Could you check a few things on this model? Use its own coordinates, in mm. Coordinates: 2 decimals unless noted, no trailing zeros. Write each loop counter-clockwise with the first axis right and the second up, starting at its lowest first coordinate (ties: lowest second). Pieces come first, ordered by that corner, then holes. Notation, with made-up numbers: (-12.75, -38) - (35.25, -38) arc R11 cw to (35.25, -22) - close; hole circle Ø7 at (16, 33.25). An arc over 180 degrees is marked (long way). Answer as a JSON object with one key per item and string values. Group by question number.
1) We'd pull the mould along Z, two halves only. Please class faces 1 (the flat face through (79, 3, -71)), 2 (the flat face through (117, 2, -115)), 3 (the flat face through (33, 2, -35)): released by +Z, released by -Z, zero draft, split by the parting line, or undercut.
2) If we section it at B-B (z = -51.5): Write out the boundary of the cut face in (x, y), plus the area to 3 significant figures.
3) Will these pins go through, and if not, where does the flat tip stop? pin 1 Ø1.5 at (y, z) = (1.5, -126) entering from +X; pin 2 Ø1 at (x, y) = (21.5, 1) entering from -Z; pin 3 Ø1.5 at (y, z) = (2, -5.5) entering from -X; pin 4 Ø1.9 at (x, z) = (100, -130) entering from +Y.
4) If we section it at A-A (x = 17): Write out the boundary of the cut face in (y, z), plus the area to 3 significant figures.
5) Please list where these lines run through material, in increasing order: line 1 along X through (y, z) = (2.7, -71.5); line 2 along X through (y, z) = (0.75, -45.5); line 3 along Z through (x, y) = (73, 2.8).
6) If we section it at C-C (y = 2.25): State how many separate pieces and enclosed holes the cut face has, plus the area to 3 significant figures.
```python
from build123d import *

# Parameters (mm, degrees)
SKETCH_1_W          = 130
SKETCH_1_H          = 140
SKETCH_1_R          = 1.6
SKETCH_1_W_2        = 24
SKETCH_1_H_2        = 112
EXTRUDE_1_DEPTH     = 3
SKETCH_2_W          = 25
SKETCH_2_H          = 25
CUT_EXTRUDE_1_DEPTH = 3
SKETCH_3_W          = 40
SKETCH_3_H          = 10
SKETCH_3_W_2        = 15.4
SKETCH_3_H_2        = 20
SKETCH_3_W_3        = 16
SKETCH_3_W_4        = 43.4
SKETCH_3_H_3        = 12
SKETCH_3_W_5        = 10
SKETCH_3_H_4        = 16
CUT_EXTRUDE_2_DEPTH = 192.07328437
FILLET_1_R          = 2


with BuildPart() as part:
    # 草图1 → 凸台-拉伸1 (new body)
    with BuildSketch(Plane(origin=(0, 0, 0), x_dir=(1, 0, 0), z_dir=(0, 1, 0))):
        with Locations((65, 70)):
            Rectangle(SKETCH_1_W, SKETCH_1_H)
        with Locations(Location((98.6, 78.5, 0), (0, 0, 270))):
            Circle(SKETCH_1_R, mode=Mode.SUBTRACT)
        with Locations(Location((80.6, 78.5, 0), (0, 0, 90))):
            Circle(SKETCH_1_R, mode=Mode.SUBTRACT)
        with Locations(Location((98.6, 51.5, 0), (0, 0, 90))):
            Circle(SKETCH_1_R, mode=Mode.SUBTRACT)
        with Locations(Location((80.6, 51.5, 0), (0, 0, 270))):
            Circle(SKETCH_1_R, mode=Mode.SUBTRACT)
        with Locations(Location((127, 85, 0), (0, 0, 270))):
            Circle(SKETCH_1_R, mode=Mode.SUBTRACT)
        with Locations(Location((113, 85, 0), (0, 0, 90))):
            Circle(SKETCH_1_R, mode=Mode.SUBTRACT)
        with Locations(Location((120, 66.4, 0), (0, 0, 270))):
            Circle(SKETCH_1_R, mode=Mode.SUBTRACT)
        with Locations(Location((120, 34.4, 0), (0, 0, 270))):
            Circle(SKETCH_1_R, mode=Mode.SUBTRACT)
        with Locations(Location((10, 34.4, 0), (0, 0, 90))):
            Circle(SKETCH_1_R, mode=Mode.SUBTRACT)
        with Locations(Location((10, 66.4, 0), (0, 0, 90))):
            Circle(SKETCH_1_R, mode=Mode.SUBTRACT)
        with Locations(Location((3, 85, 0), (0, 0, 90))):
            Circle(SKETCH_1_R, mode=Mode.SUBTRACT)
        with Locations(Location((17, 85, 0), (0, 0, 270))):
            Circle(SKETCH_1_R, mode=Mode.SUBTRACT)
        with Locations(Location((30, 130, 0), (0, 0, 270))):
            Circle(SKETCH_1_R, mode=Mode.SUBTRACT)
        with Locations(Location((100, 130, 0), (0, 0, 90))):
            Circle(SKETCH_1_R, mode=Mode.SUBTRACT)
        with Locations(Location((80.4, 82.5, 0), (0, 0, 270))):
            Circle(SKETCH_1_R, mode=Mode.SUBTRACT)
        with Locations(Location((80.4, 47.5, 0), (0, 0, 90))):
            Circle(SKETCH_1_R, mode=Mode.SUBTRACT)
        with Locations(Location((102.4, 82.5, 0), (0, 0, 270))):
            Circle(SKETCH_1_R, mode=Mode.SUBTRACT)
        with Locations(Location((102.4, 47.5, 0), (0, 0, 90))):
            Circle(SKETCH_1_R, mode=Mode.SUBTRACT)
        with Locations((65, 65)):
            Rectangle(SKETCH_1_W_2, SKETCH_1_H_2, mode=Mode.SUBTRACT)
    extrude(amount=EXTRUDE_1_DEPTH)

    # 草图2 → 切除-拉伸1 (cut)
    with BuildSketch(Plane(origin=(0, 3, 0), x_dir=(1, 0, 0), z_dir=(0, 1, 0))):
        with Locations((12.5, 127.5)):
            Rectangle(SKETCH_2_W, SKETCH_2_H)
        with Locations((12.5, 12.5)):
            Rectangle(SKETCH_2_W, SKETCH_2_H)
        with Locations((117.5, 12.5)):
            Rectangle(SKETCH_2_W, SKETCH_2_H)
        with Locations((117.5, 127.5)):
            Rectangle(SKETCH_2_W, SKETCH_2_H)
        with BuildLine():
            Line((59, 6.1), (52.8, 6.1))
            ThreePointArc((52.8, 6.1), (51.8, 7.1), (50.8, 6.1))
            Line((50.8, 6.1), (50.8, 2.9))
            ThreePointArc((50.8, 2.9), (51.8, 1.9), (52.8, 2.9))
            Line((52.8, 2.9), (59, 2.9))
            ThreePointArc((59, 2.9), (60, 1.9), (61, 2.9))
            Line((61, 2.9), (61, 6.1))
            ThreePointArc((61, 6.1), (60, 7.1), (59, 6.1))
        make_face()
        with BuildLine():
            ThreePointArc((34.6, 6.1), (33.6, 7.1), (32.6, 6.1))
            Line((32.6, 6.1), (32.6, 2.9))
            ThreePointArc((32.6, 2.9), (33.6, 1.9), (34.6, 2.9))
            Line((34.6, 2.9), (40.8, 2.9))
            ThreePointArc((40.8, 2.9), (41.8, 1.9), (42.8, 2.9))
            Line((42.8, 2.9), (42.8, 6.1))
            ThreePointArc((42.8, 6.1), (41.8, 7.1), (40.8, 6.1))
            Line((40.8, 6.1), (34.6, 6.1))
        make_face()
        with BuildLine():
            Line((77.2, 6.1), (71, 6.1))
            ThreePointArc((71, 6.1), (70, 7.1), (69, 6.1))
            Line((69, 6.1), (69, 2.9))
            ThreePointArc((69, 2.9), (70, 1.9), (71, 2.9))
            Line((71, 2.9), (77.2, 2.9))
            ThreePointArc((77.2, 2.9), (78.2, 1.9), (79.2, 2.9))
            Line((79.2, 2.9), (79.2, 6.1))
            ThreePointArc((79.2, 6.1), (78.2, 7.1), (77.2, 6.1))
        make_face()
        with BuildLine():
            Line((95.4, 6.1), (89.2, 6.1))
            ThreePointArc((89.2, 6.1), (88.2, 7.1), (87.2, 6.1))
            Line((87.2, 6.1), (87.2, 2.9))
            ThreePointArc((87.2, 2.9), (88.2, 1.9), (89.2, 2.9))
            Line((89.2, 2.9), (95.4, 2.9))
            ThreePointArc((95.4, 2.9), (96.4, 1.9), (97.4, 2.9))
            Line((97.4, 2.9), (97.4, 6.1))
            ThreePointArc((97.4, 6.1), (96.4, 7.1), (95.4, 6.1))
        make_face()
    extrude(amount=-CUT_EXTRUDE_1_DEPTH, mode=Mode.SUBTRACT)

    # 草图3 → 切除-拉伸2 (cut, through all)
    with BuildSketch(Plane(origin=(0, 3, 0), x_dir=(1, 0, 0), z_dir=(0, 1, 0))):
        with Locations((65, 130)):
            Rectangle(SKETCH_3_W, SKETCH_3_H)
        with Locations((40.7, 35)):
            Rectangle(SKETCH_3_W_2, SKETCH_3_H_2)
        with Locations((89.6, 65)):
            Rectangle(SKETCH_3_W_3, SKETCH_3_H_2)
        with Locations((103.3, 99)):
            Rectangle(SKETCH_3_W_4, SKETCH_3_H_3)
        with Locations((89.3, 35)):
            Rectangle(SKETCH_3_W_2, SKETCH_3_H_2)
        with Locations((120, 50.4)):
            Rectangle(SKETCH_3_W_5, SKETCH_3_H_4)
        with Locations((10, 50.4)):
            Rectangle(SKETCH_3_W_5, SKETCH_3_H_4)
        with Locations((40.4, 65)):
            Rectangle(SKETCH_3_W_3, SKETCH_3_H_2)
        with Locations((26.7, 99)):
            Rectangle(SKETCH_3_W_4, SKETCH_3_H_3)
    extrude(amount=-CUT_EXTRUDE_2_DEPTH, mode=Mode.SUBTRACT)

    # 圆角1
    fillet_1_edges = [part.edges().sort_by_distance(p)[0] for p in [
        (105, 1.5, -140),
        (130, 1.5, -115),
        (105, 1.5, -115),
        (105, 1.5, 0),
        (105, 1.5, -25),
        (130, 1.5, -25),
        (25, 1.5, 0),
        (0, 1.5, -25),
        (25, 1.5, -25),
        (25, 1.5, -140),
        (25, 1.5, -115),
        (0, 1.5, -115),
        (85, 1.5, -135),
        (85, 1.5, -125),
        (45, 1.5, -125),
        (45, 1.5, -135),
        (125, 1.5, -58.4),
        (125, 1.5, -42.4),
        (115, 1.5, -42.4),
        (115, 1.5, -58.4),
        (15, 1.5, -58.4),
        (15, 1.5, -42.4),
        (5, 1.5, -42.4),
        (5, 1.5, -58.4),
        (48.4, 1.5, -75),
        (48.4, 1.5, -55),
        (32.4, 1.5, -55),
        (32.4, 1.5, -75),
        (48.4, 1.5, -105),
        (48.4, 1.5, -93),
        (5, 1.5, -93),
        (5, 1.5, -105),
        (48.4, 1.5, -45),
        (48.4, 1.5, -25),
        (33, 1.5, -25),
        (33, 1.5, -45),
        (97.6, 1.5, -75),
        (97.6, 1.5, -55),
        (81.6, 1.5, -55),
        (81.6, 1.5, -75),
        (125, 1.5, -105),
        (125, 1.5, -93),
        (81.6, 1.5, -93),
        (81.6, 1.5, -105),
        (97, 1.5, -45),
        (97, 1.5, -25),
        (81.6, 1.5, -25),
        (81.6, 1.5, -45),
        (77, 1.5, -9),
        (77, 1.5, -121),
        (53, 1.5, -121),
        (53, 1.5, -9),
    ]]
    fillet(fillet_1_edges, radius=FILLET_1_R)


solid = part.part
```
Here are the results:
{
 "1": {"face 1": "zero draft", "face 2": "released by -Z", "face 3": "undercut"},
 "2": {"outline": "(0, 0) - (5, 0) - (5, 3) - (0, 3) - close; (15, 0) - (53, 0) - (53, 3) - (15, 3) - close; (77, 0) - (79, 0) - (79, 3) - (77, 3) - close; (82.2, 0) - (97, 0) - (97, 3) - (82.2, 3) - close; (100.2, 0) - (115, 0) - (115, 3) - (100.2, 3) - close; (125, 0) - (130, 0) - (130, 3) - (125, 3) - close", "area": "239 mm²"},
 "3": {"pin 1": "stops at x = 105", "pin 2": "stops at z = -115", "pin 3": "stops at x = 25", "pin 4": "passes through"},
 "4": {"outline": "(0, -115) - (3, -115) - (3, -105) - (0, -105) - close; (0, -93) - (3, -93) - (3, -86.6) - (0, -86.6) - close; (0, -83.4) - (3, -83.4) - (3, -25) - (0, -25) - close", "area": "224 mm²"},
 "5": {"line 1": "x = 0 to 32.4, 48.4 to 53, 77 to 81.6, 97.6 to 130", "line 2": "x = 0 to 5, 15 to 53, 77 to 115, 125 to 130", "line 3": "z = -140 to -135, -125 to -121, -9 to -6.1, -2.9 to 0"},
 "6": {"separate pieces": "1", "enclosed holes": "32", "area": "9,720 mm²"}
}
